The model under review builds one solid part; all positions refer to its coordinate system, in mm. A direction names the side the tool comes from. Coordinates: 2 decimals unless noted, no trailing zeros. Write each loop counter-clockwise with the first axis right and the second up, starting at its lowest first coordinate (ties: lowest second). Pieces come first, ordered by that corner, then holes. Notation, with made-up numbers: M 36.5,-35 L 85.5,-35 A20 ccw 85.5,-13 Z; hole C 61,23 d4. An arc over 180 degrees is marked long. Answer as a JSON object with one key per item and string values.
```python
from build123d import *

# Parameters (mm, degrees)
SKETCH_R             = 2
PAD_DEPTH            = 6
CYLINDER_R           = 3.7
CYLINDER_DEPTH       = 10
SKETCH001_W          = 14
SKETCH001_H          = 7.5
PAD001_DEPTH         = 12
SKETCH002_R          = 1.5
POCKET_DEPTH         = 14
BODY_PLACEMENT_ANGLE = 180


with BuildPart() as part:
    # Sketch → Pad (new body)
    with BuildSketch(Plane.XY):
        with BuildLine():
            ThreePointArc((2.9e-05, 5), (-5, 1e-05), (1e-05, -5))
            Line((1e-05, -5), (20.00001, -5))
            ThreePointArc((20.00001, -5), (25.000039, -1e-05), (20.000029, 5))
            Line((2.9e-05, 5), (20.000029, 5))
        make_face()
        Circle(SKETCH_R, mode=Mode.SUBTRACT)
        with Locations((20.000039, 0)):
            Circle(SKETCH_R, mode=Mode.SUBTRACT)
    extrude(amount=PAD_DEPTH)

    # Cylinder → Cylinder (cut)
    with BuildSketch(Plane(origin=(10, 5, 0), x_dir=(1, 0, 0), z_dir=(0, -1, 0))):
        Circle(CYLINDER_R)
    extrude(amount=CYLINDER_DEPTH, mode=Mode.SUBTRACT)

    # Sketch001 (on Face5 of Cylinder) → Pad001 (join)
    with BuildSketch(Plane(origin=(10, 5, 6), x_dir=(-1, 0, 0), z_dir=(0, 0, 1))):
        with Locations((0, 5)):
            Rectangle(SKETCH001_W, SKETCH001_H)
    extrude(amount=PAD001_DEPTH)

    # Sketch002 (on Face10 of Pad001) → Pocket (cut)
    with BuildSketch(Plane(origin=(17, 5, 0), x_dir=(0, 0, 1), z_dir=(1, 0, 0))):
        with Locations((15, 4.75)):
            Circle(SKETCH002_R)
    extrude(amount=-POCKET_DEPTH, mode=Mode.SUBTRACT)


with BuildPart() as part_1:
    # Body placement: moved
    add(part.part.rotate(Axis((0, 0, 0), (0, 1, 0)), BODY_PLACEMENT_ANGLE))


solid = part_1.part
```
(1) For pin 1 Ø1 at (y, z) = (-4, -6) entering from -X; pin 2 Ø4 at (y, z) = (1.5, -13.5) entering from -X; pin 3 Ø9.5 at (x, z) = (-10.5, -13) entering from +Y, all flat-tipped, find the tip position at first contact; note any pin that passes through.
Results list:
{"pin 1": "x = -23.57", "pin 2": "x = -17", "pin 3": "y = 3.75"}
(2) Draft analysis for pull direction X (two halves, no side actions). For faces 4 (the face through (5, 0, -3)), 5 (the face through (-25, 0, -3)), 6 (the face through (-10.1, 0.1, -3.7)), state which applies: released by +X, released by -X, zero draft, split by the parting line, or undercut.
Results list:
{"face 4": "released by +X", "face 5": "released by -X", "face 6": "undercut"}
(3) Add section C-C on z = -1.5. Give the boundary of the cut face in (x, y).
Results list:
{"outline": "M -20,-5 L -13.38,-5 L -13.38,5 L -20,5 A5 ccw Z; M -6.62,-5 L 0,-5 A5 ccw 0,5 L -6.62,5 Z; hole C -20,0 d4; hole C 0,0 d4"}
(4) Add section D-D on z = -5.25. Give the boundary of the cut face in (x, y).
Results list:
{"outline": "M -20,-5 L 0,-5 A5 ccw 0,5 L -20,5 A5 ccw Z; hole C -20,0 d4; hole C 0,0 d4"}
(5) For faces 1 (the face through (-10, 3.75, -12)), 2 (the face through (-10, -3.75, -12)), 3 (the face through (-3, 0, -12)), list the 3-axis set-ups (+Z, -Z, +X, -X, +Y, -Y) from which the entire face can be reached by the end or side of a thin tool; tool diameter is ignored.
Results list:
{"face 1": "-Z, +X, -X, +Y", "face 2": "-Z, +X, -X, -Y", "face 3": "-Z, +X, +Y, -Y"}
(6) Add section A-A on z = -15. Give the boundary of the cut face in (x, y).
Results list:
{"outline": "M -17,-3.75 L -3,-3.75 L -3,-1.25 L -17,-1.25 Z; M -17,1.75 L -3,1.75 L -3,3.75 L -17,3.75 Z"}
(7) Wall thickness on line 1 along Y through (x, z) = (-6.75, -15); line 2 along X through (y, z) = (1.25, -0.5); line 3 along X through (y, z) = (1.75, -4.25): over which ranges is each line inside the solid? List them lowest first. Write a range as from..to.
Results list:
{"line 1": "-3.75..-1.25, 1.75..3.75", "line 2": "-24.84..-21.56, -18.44..-13.67, -6.33..-1.56, 1.56..4.84", "line 3": "-24.68..-20.97, -19.03..-0.97, 0.97..4.68"}
(8) Add section B-B on x = -1. Give the boundary of the cut face in (y, z).
Results list:
{"outline": "M -5,-6 L -1.73,-6 L -1.73,0 L -5,0 Z; M 1.73,-6 L 5,-6 L 5,0 L 1.73,0 Z"}
